from build123d import *

# Parameters (mm, degrees)
SKICA1_W                 = 29.9
SKICA1_H                 = 4.4
SKICA1_W_2               = 4.4
SKICA1_H_2               = 25.5
P_IDAT_VYSUNUT_M1_DEPTH  = 0.4
ZAOBLIT3_R               = 15
ZAOBLIT4_R               = 20
SKICA2_R                 = 1.75
P_IDAT_VYSUNUT_M2_DEPTH  = 1.5
SKICA3_R                 = 1.9
P_IDAT_VYSUNUT_M3_DEPTH  = 2
ZKOSEN_1_SIZE            = 1.5
SKICA4_W                 = 3.8
SKICA4_H                 = 1
SKICA4_W_2               = 1
SKICA4_H_2               = 3.8
ODEBRAT_VYSUNUT_M1_DEPTH = 3.5


with BuildPart() as part:
    # Skica1 → Přidat vysunutím1 (new body)
    with BuildSketch(Plane.XY):
        with Locations((-7.066698514, 6.667743702)):
            Rectangle(SKICA1_W, SKICA1_H)
        with Locations((5.683301486, -8.282256298)):
            Rectangle(SKICA1_W_2, SKICA1_H_2)
    extrude(amount=P_IDAT_VYSUNUT_M1_DEPTH)

    # Zaoblit3
    zaoblit3_edges = [part.edges().sort_by_distance(p)[0] for p in [
        (3.483301486, 4.467743702, 0.2),
    ]]
    fillet(zaoblit3_edges, radius=ZAOBLIT3_R)

    # Zaoblit4
    zaoblit4_edges = [part.edges().sort_by_distance(p)[0] for p in [
        (7.883301486, 8.867743702, 0.2),
    ]]
    fillet(zaoblit4_edges, radius=ZAOBLIT4_R)

    # Skica2 → Přidat vysunutím2 (add)
    with BuildSketch(Plane.XY.offset(0.4)):
        with Locations((-15.016698514, 6.667743702)):
            Circle(SKICA2_R)
        with Locations((5.683301486, -14.032256298)):
            Circle(SKICA2_R)
    extrude(amount=P_IDAT_VYSUNUT_M2_DEPTH)

    # Skica3 → Přidat vysunutím3 (add)
    with BuildSketch(Plane.XY.offset(1.9)):
        with Locations((-15.016698514, 6.667743702)):
            Circle(SKICA3_R)
        with Locations((5.683301486, -14.032256298)):
            Circle(SKICA3_R)
    extrude(amount=P_IDAT_VYSUNUT_M3_DEPTH)

    # Zkosení1
    zkosen_1_edges = [part.edges().sort_by_distance(p)[0] for p in [
        (3.783301486, -14.032256298, 3.9),
        (-16.916698514, 6.667743702, 3.9),
    ]]
    chamfer(zkosen_1_edges, length=ZKOSEN_1_SIZE)

    # Skica4 → Odebrat vysunutím1 (cut)
    with BuildSketch(Plane.XY.offset(3.9)):
        with Locations((5.683301486, -14.032256298)):
            Rectangle(SKICA4_W, SKICA4_H)
        with Locations((-15.016698514, 6.667743702)):
            Rectangle(SKICA4_W_2, SKICA4_H_2)
    extrude(amount=-ODEBRAT_VYSUNUT_M1_DEPTH, mode=Mode.SUBTRACT)


solid = part.part
Build history of the part. All positions in model axes, mm. A direction names the side the tool comes from. Round coordinates to 2 decimals unless told otherwise and drop trailing zeros. Loops run counter-clockwise (first coordinate to the right, second up) from the corner with the lowest first, then second, coordinate; pieces in that order, holes last. Notation, with made-up numbers: (63.25, 80.5) -> (110.25, 80.5) arc R15 ccw to (110.25, 96.5) -> close; hole circle Ø8 at (24.5, 68). An arc over 180 degrees is marked (long way). One line per item, written item: value. Start each with the question number.
Q1. Two-plate mould, pull along Z, no slides. Class faces 1 (the face through (-15.517, 7, 2)), 2 (the face through (-13.267, 6.636, 1.14)), 3 (the face through (5.66, -15.22, 3.11)): released by +Z, released by -Z, zero draft, split by the parting line, or undercut.
Q2. Cut at D-D on y = -5.75. List the corners of the cut face in (x, z).
Q3. Drop flat-ended pins along their axis: pin 1 Ø1.7 at (x, z) = (5.5, 2.5) entering from -Y; pin 2 Ø6 at (x, y) = (-11.5, 3.5) entering from +Z; pin 3 Ø1 at (y, z) = (-13.5, 3) entering from -X. Give the stop position or say it passes through.
Q4. Cut at C-C on z = 3.45. List the corners of the cut face in (x, y).
Q5. 3-axis set-ups, long thin cutter, end or side, ignore diameter. For faces 4 (the face through (6, -14.532, 2)), 5 (the face through (-13.117, 6.633, 2.146)), 6 (the face through (5.65, -15.93, 2.15)), 7 (the face through (-16.916, 6.702, 2.146)), 8 (the face through (-14.517, 7, 2)): which of +Z, -Z, +X, -X, +Y, -Y reach the whole face in a straight line?
Q6. Cut at B-B on x = -20. List the corners of the cut face in (y, z), plus the area to 3 significant figures.
Q7. Cut at A-A on z = 1.2. List the corners of the cut face in (x, y), plus the area to 3 significant figures.
Q8. Probe line 1 along X through (y, z) = (6.5, 0.95); line 2 along X through (y, z) = (7, 2.9); line 3 along Z through (x, y) = (-17.25, 7). List the from-to ranges inside material, lowest first.
Computed:
1. face 1: zero draft
1. face 2: undercut
1. face 3: released by +Z
2. outline: (2.7, 0) -> (7.15, 0) -> (7.15, 0.4) -> (2.7, 0.4) -> close
3. pin 1: y = -15.93
3. pin 2: z = 2.57
3. pin 3: x = 3.96
4. outline: (-15.52, 5.98) -> (-15.52, 7.36) arc R0.85 ccw to start; (-14.52, 5.98) arc R0.85 ccw to (-14.52, 7.36) -> close; (5, -14.53) arc R0.85 ccw to (6.37, -14.53) -> close; (5, -13.53) -> (6.37, -13.53) arc R0.85 ccw to start
5. face 4: +Z, +X, -X
5. face 5: +Z, +X
5. face 6: +Z, -Y
5. face 7: +Z, -X
5. face 8: +Z, +Y, -Y
6. outline: (4.47, 0) -> (8.87, 0) -> (8.87, 0.4) -> (4.47, 0.4) -> close
6. area: 1.76 mm²
7. outline: (-15.52, 4.99) -> (-15.52, 8.34) arc R1.75 ccw to start; (-14.52, 4.99) arc R1.75 ccw to (-14.52, 8.34) -> close; (4.01, -14.53) arc R1.75 ccw to (7.36, -14.53) -> close; (4.01, -13.53) -> (7.36, -13.53) arc R1.75 ccw to start
7. area: 12.3 mm²
8. line 1: -16.76 to -15.52, -14.52 to -13.27
8. line 2: -16.38 to -15.52, -14.52 to -13.66
8. line 3: 0 to 0.4
